The model under review builds one solid part; all positions refer to its coordinate system, in mm. A direction names the side the tool comes from. Round coordinates to 2 decimals unless told otherwise and drop trailing zeros. Loops run counter-clockwise (first coordinate to the right, second up) from the corner with the lowest first, then second, coordinate; pieces in that order, holes last. Notation, with made-up numbers: M 64.5,50.5 L 119.5,50.5 A13 ccw 119.5,58.5 Z; hole C 45.25,65 d7. An arc over 180 degrees is marked long. One line per question, with ' | ' between items.
from build123d import *

# Parameters (mm, degrees)
CUT_EXTRUDE2_START  = -30
CUT_EXTRUDE2_DEPTH  = 30
SKETCH6_R           = 8
BOSS_EXTRUDE1_DEPTH = 10
CUT_EXTRUDE3_DEPTH  = 15
FILLET1_R           = 1
SKETCH8_R           = 2.5
CUT_EXTRUDE4_DEPTH  = 1


with BuildPart() as part:
    # Sketch2 → Revolve2 (revolve)
    with BuildSketch(Plane(origin=(0, 0, 0), x_dir=(1, 0, 0), z_dir=(0, 1, 0)), mode=Mode.PRIVATE) as revolve2_sk:
        Polygon((0, -40), (8, -40), (8, -10), (12.5, -10), (12.5, 25), (8, 25), (8, 40), (0, 40), align=None)
    revolve(revolve2_sk.sketch.rotate(Axis((0, 0, -364.100348117), (0, 0, 1)), 180), axis=Axis((0, 0, -364.100348117), (0, 0, 1)))

    # Sketch4 → Cut-Extrude2 (cut)
    with BuildSketch(Plane.XY.offset(40).offset(CUT_EXTRUDE2_START)):
        with BuildLine():
            Line((-6.61, 1.39), (-7.878318348, 1.39))
            ThreePointArc((-7.878318348, 1.39), (-8, 0), (-7.878318348, -1.39))
            Line((-7.878318348, -1.39), (-6.61, -1.39))
            Line((-6.61, -1.39), (-6.61, 1.39))
        make_face()
    extrude(amount=CUT_EXTRUDE2_DEPTH, mode=Mode.SUBTRACT)

    # Sketch6 → Boss-Extrude1 (add)
    with BuildSketch(Plane.XY.offset(40)):
        with Locations(Location((0, 0, 0), (0, 0, 190.005924043))):
            Circle(SKETCH6_R)
    extrude(amount=BOSS_EXTRUDE1_DEPTH)

    # Sketch7 → Cut-Extrude3 (cut)
    with BuildSketch(Plane(origin=(0, 0, -40), x_dir=(-1, 0, 0), z_dir=(0, 0, -1))):
        with BuildLine():
            Line((-4, 6.92820323), (-4, -6.92820323))
            ThreePointArc((-4, -6.92820323), (-8, 0), (-4, 6.92820323))
        make_face()
        with BuildLine():
            Line((4, 6.92820323), (4, -6.92820323))
            ThreePointArc((4, -6.92820323), (8, 0), (4, 6.92820323))
        make_face()
    extrude(amount=-CUT_EXTRUDE3_DEPTH, mode=Mode.SUBTRACT)

    # Fillet1
    fillet1_edges = [part.edges().sort_by_distance(p)[0] for p in [
        (4, 6.92820323, -32.5),
        (4, -6.92820323, -32.5),
        (-4, -6.92820323, -32.5),
        (-4, 6.92820323, -32.5),
    ]]
    fillet(fillet1_edges, radius=FILLET1_R)

    # Sketch8 → Cut-Extrude4 (cut)
    with BuildSketch(Plane.ZY.offset(4)):
        with Locations((-32.5, 0)):
            Circle(SKETCH8_R)
    extrude(amount=-CUT_EXTRUDE4_DEPTH, mode=Mode.SUBTRACT)


solid = part.part
1) Add section C-C on x = 0. State the section outline as (y, z) points.
Output values:
outline: M -12.5,-25 L -8,-25 L -8,-40 L 8,-40 L 8,-25 L 12.5,-25 L 12.5,10 L 8,10 L 8,50 L -8,50 L -8,10 L -12.5,10 Z
2) Add section A-A on y = 0. State the section outline as (x, z) points, then the cut area to 3 significant figures.
Output values:
outline: M -12.5,-25 L -4,-25 L -4,-30 L -3,-30 L -3,-35 L -4,-35 L -4,-40 L 4,-40 L 4,-25 L 12.5,-25 L 12.5,10 L 8,10 L 8,50 L -8,50 L -8,40 L -6.61,40 L -6.61,10 L -12.5,10 Z | area: 1,590 mm²
3) Insertion check: P1, Ø1, axis at x = 1.5, y = 10, coming from the +Z side; P2, Ø0.7, axis at x = -7.5, y = -0.5, coming from the -Z side; P3, Ø1, axis at x = -7.5, z = 17.5, coming from the -Y side. Each pin has a flat end and moves straight along its axis. Give the tip position at first contact, or say it passes through.
Output values:
P1: stops at z = 10 | P2: stops at z = -25 | P3: stops at y = -3.87
4) For line 1 (X direction, y = 5.75, z = -26); line 2 (Z direction, x = -3.25, y = -1.25); line 3 (Y direction, x = -3.25, z = -32.5), list the stretches that pass through material, from the lowest coordinate up.
Output values:
line 1: x = -4 to 4 | line 2: z = -40 to -34.67, -30.33 to 50 | line 3: y = -7.31 to -2.5, 2.5 to 7.31
5) Add section D-D on z = 5. State the section outline as (x, y) points, then the cut area to 3 significant figures.
Output values:
outline: C 0,0 d25 | area: 491 mm²
6) Add section B-B on z = -32.5. State the section outline as (x, y) points.
Output values:
outline: M -4,-6.32 A1 ccw -3.43,-7.23 A8 ccw 3.43,-7.23 A1 ccw 4,-6.32 L 4,6.32 A1 ccw 3.43,7.23 A8 ccw -3.43,7.23 A1 ccw -4,6.32 L -4,2.5 L -3,2.5 L -3,-2.5 L -4,-2.5 Z
7) Machinability: for faces 4 (the flat face through (-5, 0, -25)), 5 (the cylindrical face through (0, -8, -33)), 6 (the flat face through (-4, 3, -33)), 7 (the cylindrical face through (-3.5, 0.1, -35)), 8 (the flat face through (0, 0, 50)), which of the approach directions +Z, -Z, +X, -X, +Y, -Y give a long, thin tool a straight path to every point of the face, cutting with its end or side? Answer none if there is none.
Output values:
face 4: -Z | face 5: -Z, -Y | face 6: -Z, -X, +Y, -Y | face 7: -X | face 8: +Z, +X, -X, +Y, -Y
8) Mouldability with a two-part tool opening along Y and no side actions: class faces 1 (the cylindrical face through (0, 8, -33)), 2 (the flat face through (-6.61, 0, 25)), 3 (the flat face through (4, 0, -33)) as +Y half, -Y half, draft (parallel to the pull), parting line (faces both ways), or undercut.
Output values:
face 1: +Y half | face 2: undercut | face 3: draft
